Autodesk Inventor part; units mm, degrees
ref_plane "Arbeitsebene1" through (0, 0, 10) normal (0, 0, 1) x (1, 0, 0)
ref_plane "Arbeitsebene3" through (0, 0, 50) normal (0, 0, 1) x (1, 0, 0)
ref_plane "Arbeitsebene4" through (0, 0, 130) normal (0, 0, 1) x (1, 0, 0)
sketch "Skizze1" plane through (0, 0, 0) normal (0, 0, 1) x (1, 0, 0)
  circle A0 centre (0, 0) radius 30
  circle A1 centre (0, 0) radius 13.5
  circle A2 centre (0, 0) radius 9.5
  circle A3 centre (0, 0) radius 23.25 construction
  line L0 (0, 0) -> (0, 23.25) construction
  line L1 (0, 0) -> (0, 30) construction
  point P0 (-23.25, 0)
  point P1 (0, -23.25)
  point P2 (23.25, 0)
  dimension "d3" = 30
  dimension "d4" = 46.5
  dimension "d0" = 4
  dimension "d1" = 27
  dimension "d7" = 360
  dimension "d99" = 0
extrude "Extrusion1" add sketch "Skizze1" along normal blind 16.5 contours A0 | A1
extrude "Extrusion2" add sketch "Skizze1" against normal blind 2.6 contours A1
sketch "Skizze2" plane through (0, 0, 16.5) normal (0, 0, 1) x (1, 0, 0)
  point P0 (0, 0)
  point P1 (0, 23.25)
  point P2 (23.25, 0)
  point P3 (0, -23.25)
  point P4 (-23.25, 0)
hole "Bohrung1" at (0, 23.25, 16.5) at (23.25, 0, 16.5) at (0, -23.25, 16.5) at (-23.25, 0, 16.5) direction (0, 0, -1) diameter 4.134 end through all
ref_plane "Arbeitsebene1" through (0, 0, 10) normal (0, 0, 1) x (1, 0, 0)
sketch "Skizze10" plane through (0, 0, 16.5) normal (0, 0, 1) x (1, 0, 0)
  line L0 (-30, 20) -> (30, 20)
  line L1 (30, 20) -> (30, -20)
  line L2 (30, -20) -> (-30, -20)
  line L3 (-30, -20) -> (-30, 20)
  line L4 (-30, 20) -> (30, -20) construction
  line L5 (30, 20) -> (-30, -20) construction
  circle A0 centre (0, 0) radius 30
  circle A1 centre (-23.25, 0) radius 2.067 construction
  circle A2 centre (0, -23.25) radius 2.067 construction
  line L6 (-20, 0) -> (20, 0) construction
  circle A3 centre (0, 0) radius 30
  line L7 (0, 42) -> (0, -42) construction
  line L8 (-17.5, 10) -> (17.5, 10) construction
  line L9 (17.5, 10) -> (17.5, -10) construction
  line L10 (17.5, -10) -> (-17.5, -10) construction
  line L11 (-17.5, -10) -> (-17.5, 10) construction
  line L12 (-17.5, 10) -> (17.5, -10) construction
  line L13 (17.5, 10) -> (-17.5, -10) construction
  point P0 (-22.3607, 20)
  point P1 (-22.3607, -20)
  point P2 (22.3607, -20)
  point P3 (22.3607, 20)
  point P4 (30, 0)
  point P5 (-30, 0)
  dimension "d81" = 40
  dimension "ItemFixation_HoleDia" = 40
  dimension "d102" = 20
  dimension "d103" = 35
extrude "Extrusion7" cut sketch "Skizze10" against normal blind 5 contours L0 A0 L3 | L0 A0 L2 | A0 L2 L3 | L0 L1 A0 | L1 L2 A0
sketch "Skizze11" plane through (0, 0, 0) normal (0, 0, -1) x (-1, 0, 0)
  point P0 (0, 0)
  point P1 (-17.5, 10)
  point P2 (-17.5, -10)
  point P3 (17.5, -10)
  point P4 (17.5, 10)
  dimension "MainAxis_Schluesselweite" = 24
  dimension "d46" = 1
  dimension "d52" = 32
hole "Bohrung4" at (17.5, 10, 0) at (17.5, -10, 0) at (-17.5, -10, 0) at (-17.5, 10, 0) direction (0, 0, 1) diameter 4.5 end through all countersink diameter 9.4 countersink angle 90
chamfer "Fase3" distance 1 angle 45 4 edges at (22.3607, 20, 14) (-22.3607, 20, 14) (-22.3607, -20, 14) (22.3607, -20, 14)
sketch "Skizze8" plane through (12, -16, 160) normal (1, 0, 0) x (0, 0, -1)
  line L0 (30, -26) -> (30, 58) construction
  line L1 (-32.52, 16) -> (195.12, 16) construction
  point P0 (160, 16)
  point P1 (30, 16)
  dimension "Flansch_ParralelMech_FlatPart_Width" = 140
sketch "Skizze4" plane through (0, 0, 0) normal (1, 0, 0) x (0, 1, 0)
  line L0 (9.5, -2.6) -> (-9.5, -2.6) construction
  line L1 (0, 200.32) -> (0, -36.42) construction
  line L2 (-9.5, 16.5) -> (-9.5, -2.6) construction
  line L3 (9.5, 16.5) -> (9.5, -2.6) construction
  line L4 (-9.5, 16.5) -> (9.5, 16.5) construction
  line L5 (-9.5, 2.4) -> (9.5, 2.4)
  line L6 (-9.5, 2.4) -> (-9.5, 16.5)
  line L7 (-9.5, 16.5) -> (-20, 16.5)
  line L8 (-20, 16.5) -> (-20, 166.5)
  line L9 (-20, 166.5) -> (20, 166.5)
  line L10 (20, 16.5) -> (9.5, 16.5)
  line L11 (9.5, 16.5) -> (9.5, 2.4)
  line L12 (20, 166.5) -> (20, 16.5)
  line L13 (0, 2.4) -> (0, 166.5)
  point P0 (0, 0)
  dimension "d27" = 5
  dimension "d31" = 150
  dimension "d33" = 40
sketch "Skizze7" plane through (0, 0, 50) normal (0, 0, 1) x (1, 0, 0)
  line L0 (-12, 16) -> (-12, -16) construction
  line L1 (-12, 15) -> (-3, 15)
  line L2 (-3, 15) -> (-3, 11.425)
  line L3 (-3, 11.425) -> (3, 11.425)
  line L4 (3, 11.425) -> (3, 15)
  line L5 (3, 15) -> (12, 15)
  line L6 (-12, 0) -> (-12, 15)
  line L7 (0, -16) -> (0, 16) construction
  line L8 (12, -16) -> (12, 16) construction
  line L9 (12, 15) -> (12, 0)
  line L10 (-12, 0) -> (12, 0)
  line L11 (-42, 0) -> (42, 0) construction
  point P0 (0, 11.425)
  point P1 (-12, -7.2111)
  point P2 (12, 7.2111)
  dimension "d51" = 9
  dimension "d63" = 30
  dimension "d64" = 22.85
equation "\"d3\" = Flansch_FemalePart_OuterDia"
equation "\"d4\" = Flansch_FemalePart_HoleDia"
equation "\"d1\" = Flansch_Klemmdeckelausnahme_Dia"
equation "\"d102\" = Item40x40_TrackDistance"
equation "\"d33\" = d28"
equation "\"Total_Bearing_Hole_Dist\" = 80"
properties part number "Flansch_FemalePart_MainAxis_HeadConnectorBase_V2.1_Item40x40" material "Edelstahl"
Geometry check sheet. Reference: the model listing, model coordinates, mm. A direction names the side the tool comes from. Round coordinates to 2 decimals unless told otherwise and drop trailing zeros. Write each loop counter-clockwise with the first axis right and the second up, starting at its lowest first coordinate (ties: lowest second). Pieces come first, ordered by that corner, then holes. Notation, with made-up numbers: (6, 17) -> (41, 17) arc R24 cw to (41, 45) -> close; hole circle Ø7 at (24, 29). An arc over 180 degrees is marked (long way). Put each result on its own line as item: value.
1) Release check for a two-part mould opening along X. For faces 3 (the face through (15.154, 9.479, 2.297)), 4 (the face through (-2.93, -13.18, -1.28)), 5 (the face through (0, -20, 14)) record: pulls with the +X half, pulls with the -X half, needs draft (parallel to the pull), parting line crosses it, or undercut.
Recorded:
face 3: undercut
face 4: parting line crosses it
face 5: needs draft
2) Cross-section at B-B, the plane y = 0. Enter the section's corners in (x, z), plus the area to 3 significant figures.
Recorded:
outline: (-30, 0) -> (-25.32, 0) -> (-25.32, 11.5) -> (-30, 11.5) -> close; (-21.18, 0) -> (-13.5, 0) -> (-13.5, -2.6) -> (-9.5, -2.6) -> (-9.5, 11.5) -> (-21.18, 11.5) -> close; (9.5, -2.6) -> (13.5, -2.6) -> (13.5, 0) -> (21.18, 0) -> (21.18, 11.5) -> (9.5, 11.5) -> close; (25.32, 0) -> (30, 0) -> (30, 11.5) -> (25.32, 11.5) -> close
area: 397 mm2
3) Thickness scan on probe 1 along Y at (x, z) = (17.5, 9.75); probe 2 along X at (y, z) = (-10, 7.25); probe 3 along Y at (x, z) = (-18.5, 3.75). Record the ranges inside material, lowest first. Write a range as from..to.
Recorded:
probe 1: y = -24.37..-12.25, -7.75..7.75, 12.25..24.37
probe 2: x = -28.28..-19.75, -15.25..15.25, 19.75..28.28
probe 3: y = -23.62..-12.02, -7.98..7.98, 12.02..23.62
4) Cross-section at A-A, the plane z = 15.5. Enter the section's corners in (x, y), plus the area to 3 significant figures.
Recorded:
outline: (-21.68, -20.73) arc R30 ccw to (21.68, -20.73) -> (21.36, -20) -> (-21.36, -20) -> close; (-21.68, 20.73) -> (-21.36, 20) -> (21.36, 20) -> (21.68, 20.73) arc R30 ccw to start; hole circle Ø4.13 at (0, -23.25); hole circle Ø4.13 at (0, 23.25)
area: 591 mm2
5) Cross-section at D-D, the plane x = 0. Enter the section's corners in (y, z).
Recorded:
outline: (-30, 0) -> (-25.32, 0) -> (-25.32, 16.5) -> (-30, 16.5) -> close; (-21.18, 0) -> (-13.5, 0) -> (-13.5, -2.6) -> (-9.5, -2.6) -> (-9.5, 11.5) -> (-20, 11.5) -> (-20, 16.5) -> (-21.18, 16.5) -> close; (9.5, -2.6) -> (13.5, -2.6) -> (13.5, 0) -> (21.18, 0) -> (21.18, 16.5) -> (20, 16.5) -> (20, 11.5) -> (9.5, 11.5) -> close; (25.32, 0) -> (30, 0) -> (30, 16.5) -> (25.32, 16.5) -> close
6) Access from +Z, -Z, +X, -X, +Y, -Y to the whole of each face (thin tool, end or side, straight path). Record for faces 1 (the face through (21.5, -1.1, 5.7)), 2 (the face through (-14, 0, 0)).
Recorded:
face 1: +Z, -Z
face 2: -Z
7) Cross-section at C-C, the plane z = 1.25. Give the number of separate pieces and of enclosed holes in the cut face, plus the area to 3 significant figures.
Recorded:
separate pieces: 1
enclosed holes: 9
area: 2,340 mm2
8) Depth check by flat-ended pin: P1, Ø10, axis at y = 23, z = 3.5, coming from the -X side; P2, Ø6.5, axis at x = -23.25, y = 0, coming from the +Z side; P3, Ø3, axis at x = 3, z = -0.5, coming from the -Y side. Enter the tip coordinate at first touch or a pass-through.
Recorded:
P1: stops at x = -24
P2: stops at z = 11.5
P3: stops at y = -29.96
